Geometry check sheet. Reference: the model listing, model coordinates, mm. A direction names the side the tool comes from. Give positions to 0.01 mm unless a question says otherwise; leave off trailing zeros. Loops run counter-clockwise (first coordinate to the right, second up) from the corner with the lowest first, then second, coordinate; pieces in that order, holes last. Notation, with made-up numbers: (-8.5, 1.25) -> (4.5, 1.25) arc R20 ccw to (4.5, 31.25) -> close; hole circle Ø5 at (85.25, 18.25). An arc over 180 degrees is marked (long way). Answer as a JSON object with one key per item and string values.
Autodesk Inventor part; units mm, degrees
ref_plane "YZ Plane" through (0, 0, 0) normal (1, 0, 0) x (0, 1, 0)
ref_plane "XZ Plane" through (0, 0, 0) normal (0, 1, 0) x (-1, 0, 0)
ref_plane "XY Plane" through (0, 0, 0) normal (0, 0, 1) x (1, 0, 0)
sketch "Sketch2" plane through (0, 0, 0) normal (0, 0, 1) x (1, 0, 0)
  line L0 (-38.1, 105.1577) -> (50.8, 105.1577)
  line L1 (50.8, 105.1577) -> (50.8, 16.2577)
  line L2 (50.8, 16.2577) -> (-38.1, 16.2577)
  line L3 (-38.1, 16.2577) -> (-38.1, 105.1577)
  point P0 (0, 0)
  dimension "d45" = 88.9
  dimension "d46" = 88.9
extrude "Extrusion1" add sketch "Sketch2" along normal blind 2.54
sketch "Sketch3" plane through (0, 0, 0) normal (0, 0, -1) x (-1, 0, 0)
  circle A0 centre (-43.18, 97.5377) radius 4.0005
  line L0 (-50.8, 16.2577) -> (-50.8, 105.1577)
  line L1 (-50.8, 105.1577) -> (38.1, 105.1577)
  circle A1 centre (-43.18, 97.5377) radius 5.2705
  line L2 (38.1, 105.1577) -> (38.1, 16.2577)
  line L3 (38.1, 16.2577) -> (-50.8, 16.2577)
  circle A2 centre (-43.18, 84.8377) radius 5.2705
  circle A3 centre (-30.48, 97.5377) radius 5.2705
  circle A4 centre (-30.48, 84.8377) radius 5.2705
  circle A5 centre (-17.78, 97.5377) radius 5.2705
  circle A6 centre (-17.78, 84.8377) radius 5.2705
  line L4 (-45.1739, 77.2092) -> (-41.1861, 77.2092)
  line L5 (-41.1861, 77.2092) -> (-41.1861, 74.1358)
  line L6 (-41.1861, 74.1358) -> (-45.1739, 74.1358)
  line L7 (-45.1739, 74.1358) -> (-45.1739, 77.2092)
  line L8 (-45.1739, 77.2092) -> (-41.1861, 74.1358) construction
  line L9 (-41.1861, 77.2092) -> (-45.1739, 74.1358) construction
  line L10 (-45.9813, 73.5135) -> (-40.3787, 73.5135)
  line L11 (-40.3787, 73.5135) -> (-40.3787, 77.8315)
  line L12 (-40.3787, 77.8315) -> (-45.9813, 77.8315)
  line L13 (-45.9813, 77.8315) -> (-45.9813, 73.5135)
  line L14 (-45.9813, 73.5135) -> (-40.3787, 77.8315) construction
  line L15 (-40.3787, 73.5135) -> (-45.9813, 77.8315) construction
  circle A7 centre (-30.48, 97.5377) radius 4.1255
  circle A8 centre (-17.78, 97.5377) radius 4.2505
  circle A9 centre (-43.18, 84.8377) radius 4.3755
  circle A10 centre (-30.48, 84.8377) radius 4.5005
  circle A11 centre (-17.78, 84.8377) radius 4.6255
  line L16 (-32.7587, 77.8315) -> (-38.3613, 77.8315)
  line L17 (-38.3613, 77.8315) -> (-38.3613, 73.5135)
  line L18 (-38.3613, 73.5135) -> (-32.7587, 73.5135)
  line L19 (-32.7587, 73.5135) -> (-32.7587, 77.8315)
  line L20 (-25.1387, 77.8315) -> (-30.7413, 77.8315)
  line L21 (-30.7413, 77.8315) -> (-30.7413, 73.5135)
  line L22 (-30.7413, 73.5135) -> (-25.1387, 73.5135)
  line L23 (-25.1387, 73.5135) -> (-25.1387, 77.8315)
  line L24 (-17.5187, 77.8315) -> (-23.1213, 77.8315)
  line L25 (-23.1213, 77.8315) -> (-23.1213, 73.5135)
  line L26 (-23.1213, 73.5135) -> (-17.5187, 73.5135)
  line L27 (-17.5187, 73.5135) -> (-17.5187, 77.8315)
  line L28 (-9.8987, 77.8315) -> (-15.5013, 77.8315)
  line L29 (-15.5013, 77.8315) -> (-15.5013, 73.5135)
  line L30 (-15.5013, 73.5135) -> (-9.8987, 73.5135)
  line L31 (-9.8987, 73.5135) -> (-9.8987, 77.8315)
  line L32 (-37.6789, 74.0108) -> (-33.4411, 74.0108)
  line L33 (-33.4411, 74.0108) -> (-33.4411, 77.3342)
  line L34 (-33.4411, 77.3342) -> (-37.6789, 77.3342)
  line L35 (-37.6789, 77.3342) -> (-37.6789, 74.0108)
  line L36 (-37.6789, 74.0108) -> (-33.4411, 77.3342) construction
  line L37 (-33.4411, 74.0108) -> (-37.6789, 77.3342) construction
  line L38 (-30.1839, 73.8858) -> (-25.6961, 73.8858)
  line L39 (-25.6961, 73.8858) -> (-25.6961, 77.4592)
  line L40 (-25.6961, 77.4592) -> (-30.1839, 77.4592)
  line L41 (-30.1839, 77.4592) -> (-30.1839, 73.8858)
  line L42 (-30.1839, 73.8858) -> (-25.6961, 77.4592) construction
  line L43 (-25.6961, 73.8858) -> (-30.1839, 77.4592) construction
  line L44 (-22.6889, 73.7608) -> (-17.9511, 73.7608)
  line L45 (-17.9511, 73.7608) -> (-17.9511, 77.5842)
  line L46 (-17.9511, 77.5842) -> (-22.6889, 77.5842)
  line L47 (-22.6889, 77.5842) -> (-22.6889, 73.7608)
  line L48 (-22.6889, 73.7608) -> (-17.9511, 77.5842) construction
  line L49 (-17.9511, 73.7608) -> (-22.6889, 77.5842) construction
  line L50 (-45.1739, 73.4552) -> (-41.1861, 73.4552)
  line L51 (-41.1861, 73.4552) -> (-41.1861, 74.8164)
  line L52 (-41.1861, 74.8164) -> (-45.1739, 74.8164)
  line L53 (-45.1739, 74.8164) -> (-45.1739, 73.4552)
  line L54 (-45.1739, 73.4552) -> (-41.1861, 74.8164) construction
  line L55 (-41.1861, 73.4552) -> (-45.1739, 74.8164) construction
  point P0 (0, 0)
  point P1 (-43.18, 75.6725)
  point P2 (-43.18, 75.6725)
  point P3 (-35.56, 75.6725)
  point P4 (-27.94, 75.6725)
  point P5 (-20.32, 75.6725)
  point P6 (-12.7, 75.6725)
  point P7 (-43.18, 74.1358)
  dimension "d49" = 7.62
  dimension "d50" = 7.62
  dimension "d51" = 1.27
  dimension "d56" = 12.7
  dimension "d59" = 12.7
  dimension "d64" = 3.9878
  dimension "d65" = 3.0734
  dimension "d66" = 9.1652
  dimension "d67" = 2.159
  dimension "d77" = 8.001
  dimension "d78" = 8.251
  dimension "d80" = 8.501
  dimension "d81" = 8.751
  dimension "d82" = 9.001
  dimension "d83" = 9.251
  dimension "d90" = 7.62
  dimension "d95" = 4.2378
  dimension "d96" = 4.4878
  dimension "d97" = 4.7378
  dimension "d98" = 3.3234
  dimension "d99" = 3.5734
sketch "Sketch4" plane through (0, 0, 0) normal (0, 0, -1) x (-1, 0, 0)
  line L0 (-50.8, 105.1577) -> (38.1, 105.1577)
  line L1 (-50.8, 16.2577) -> (-50.8, 105.1577)
  line L2 (-50.8, 105.1577) -> (-48.5295, 105.1577)
  line L3 (-48.5295, 105.1577) -> (-48.5295, 103.1024)
  line L4 (-48.5295, 103.1024) -> (-50.8, 103.1024)
  line L5 (-50.8, 103.1024) -> (-50.8, 105.1577)
  point P0 (0, 0)
extrude "Extrusion4" cut sketch "Sketch3" against normal blind 9.001 contours A0 | A7 | A8 | A9 | A10 | A11
sketch "Sketch5" plane through (0, 0, 0) normal (0, 0, -1) x (-1, 0, 0)
  line L0 (-45.1739, 39.1092) -> (-41.1861, 39.1092)
  line L1 (-41.1861, 39.1092) -> (-41.1861, 36.0358)
  line L2 (-41.1861, 36.0358) -> (-45.1739, 36.0358)
  line L3 (-45.1739, 36.0358) -> (-45.1739, 39.1092)
  line L4 (-45.1739, 39.1092) -> (-41.1861, 36.0358) construction
  line L5 (-41.1861, 39.1092) -> (-45.1739, 36.0358) construction
  line L6 (-45.9813, 35.4135) -> (-40.3787, 35.4135)
  line L7 (-40.3787, 35.4135) -> (-40.3787, 39.7315)
  line L8 (-40.3787, 39.7315) -> (-45.9813, 39.7315)
  line L9 (-45.9813, 39.7315) -> (-45.9813, 35.4135)
  line L10 (-45.9813, 35.4135) -> (-40.3787, 39.7315) construction
  line L11 (-40.3787, 35.4135) -> (-45.9813, 39.7315) construction
  line L12 (-32.7587, 39.7315) -> (-38.3613, 39.7315)
  line L13 (-38.3613, 39.7315) -> (-38.3613, 35.4135)
  line L14 (-38.3613, 35.4135) -> (-32.7587, 35.4135)
  line L15 (-32.7587, 35.4135) -> (-32.7587, 39.7315)
  line L16 (-25.1387, 39.7315) -> (-30.7413, 39.7315)
  line L17 (-30.7413, 39.7315) -> (-30.7413, 35.4135)
  line L18 (-30.7413, 35.4135) -> (-25.1387, 35.4135)
  line L19 (-25.1387, 35.4135) -> (-25.1387, 39.7315)
  line L20 (-17.5187, 39.7315) -> (-23.1213, 39.7315)
  line L21 (-23.1213, 39.7315) -> (-23.1213, 35.4135)
  line L22 (-23.1213, 35.4135) -> (-17.5187, 35.4135)
  line L23 (-17.5187, 35.4135) -> (-17.5187, 39.7315)
  line L24 (-9.8987, 39.7315) -> (-15.5013, 39.7315)
  line L25 (-15.5013, 39.7315) -> (-15.5013, 35.4135)
  line L26 (-15.5013, 35.4135) -> (-9.8987, 35.4135)
  line L27 (-37.6789, 35.9108) -> (-33.4411, 35.9108)
  line L28 (-33.4411, 35.9108) -> (-33.4411, 39.2342)
  line L29 (-33.4411, 39.2342) -> (-37.6789, 39.2342)
  line L30 (-37.6789, 39.2342) -> (-37.6789, 35.9108)
  line L31 (-37.6789, 35.9108) -> (-33.4411, 39.2342) construction
  line L32 (-33.4411, 35.9108) -> (-37.6789, 39.2342) construction
  line L33 (-30.1839, 35.7858) -> (-25.6961, 35.7858)
  line L34 (-25.6961, 35.7858) -> (-25.6961, 39.3592)
  line L35 (-25.6961, 39.3592) -> (-30.1839, 39.3592)
  line L36 (-30.1839, 39.3592) -> (-30.1839, 35.7858)
  line L37 (-30.1839, 35.7858) -> (-25.6961, 39.3592) construction
  line L38 (-25.6961, 35.7858) -> (-30.1839, 39.3592) construction
  line L39 (-22.6889, 35.6608) -> (-17.9511, 35.6608)
  line L40 (-17.9511, 35.6608) -> (-17.9511, 39.4842)
  line L41 (-17.9511, 39.4842) -> (-22.6889, 39.4842)
  line L42 (-22.6889, 39.4842) -> (-22.6889, 35.6608)
  line L43 (-22.6889, 35.6608) -> (-17.9511, 39.4842) construction
  line L44 (-17.9511, 35.6608) -> (-22.6889, 39.4842) construction
  line L45 (-45.1516, 35.2931) -> (-41.1861, 36.7869) construction
  line L46 (-41.1861, 35.3552) -> (-45.1739, 36.7164) construction
  line L47 (-44.9867, 35.3552) -> (-41.3733, 35.3552)
  line L48 (-41.3733, 35.3552) -> (-41.3733, 36.7164)
  line L49 (-41.3733, 36.7164) -> (-44.9867, 36.7164)
  line L50 (-44.9867, 36.7164) -> (-44.9867, 35.3552)
  line L51 (-44.9867, 35.3552) -> (-41.3733, 36.7164) construction
  line L52 (-41.3733, 35.3552) -> (-44.9867, 36.7164) construction
  line L53 (-37.5427, 35.3747) -> (-33.5773, 35.3747)
  line L54 (-33.5773, 35.3747) -> (-33.5773, 36.447)
  line L55 (-33.5773, 36.447) -> (-37.5427, 36.447)
  line L56 (-37.5427, 36.447) -> (-37.5427, 35.3747)
  line L57 (-37.5427, 35.3747) -> (-33.5773, 36.447) construction
  line L58 (-33.5773, 35.3747) -> (-37.5427, 36.447) construction
  line L59 (-30.0124, 35.3468) -> (-25.8676, 35.3468)
  line L60 (-25.8676, 35.3468) -> (-25.8676, 36.2248)
  line L61 (-25.8676, 36.2248) -> (-30.0124, 36.2248)
  line L62 (-30.0124, 36.2248) -> (-30.0124, 35.3468)
  line L63 (-30.0124, 35.3468) -> (-25.8676, 36.2248) construction
  line L64 (-25.8676, 35.3468) -> (-30.0124, 36.2248) construction
  line L65 (-22.4558, 35.2013) -> (-18.1842, 35.2013)
  line L66 (-18.1842, 35.2013) -> (-18.1842, 36.1203)
  line L67 (-18.1842, 36.1203) -> (-22.4558, 36.1203)
  line L68 (-22.4558, 36.1203) -> (-22.4558, 35.2013)
  line L69 (-22.4558, 35.2013) -> (-18.1842, 36.1203) construction
  line L70 (-18.1842, 35.2013) -> (-22.4558, 36.1203) construction
  point P0 (0, 0)
  point P1 (-43.18, 37.5725)
  point P2 (-43.18, 37.5725)
  point P3 (-35.56, 37.5725)
  point P4 (-27.94, 37.5725)
  point P5 (-20.32, 37.5725)
  point P6 (-12.7, 37.5725)
  point P7 (-43.18, 36.0358)
  point P8 (-35.56, 35.9108)
  point P9 (-27.94, 35.7858)
  point P10 (-20.32, 35.6608)
  point P11 (-22.4558, 35.4135)
  point P12 (-22.4558, 35.6608)
  point P13 (-18.1842, 35.6608)
  point P14 (-18.1842, 35.4135)
  point P15 (-30.0124, 35.4135)
  point P16 (-30.0124, 35.7858)
  point P17 (-25.8676, 35.7858)
  point P18 (-25.8676, 35.4135)
  point P19 (-37.5427, 35.4135)
  point P20 (-37.5427, 35.9108)
  point P21 (-33.5773, 35.9108)
  point P22 (-33.5773, 35.4135)
  point P23 (-44.9867, 35.4135)
  point P24 (-44.9867, 36.0358)
  point P25 (-41.3733, 36.0358)
  point P26 (-41.3733, 35.4135)
  dimension "d102" = 3.0734
  dimension "d103" = 2.159
  dimension "d104" = 7.62
  dimension "d105" = 4.2378
  dimension "d106" = 4.4878
  dimension "d107" = 4.7378
  dimension "d108" = 3.3234
  dimension "d109" = 3.5734
extrude "Extrusion5" add sketch "Sketch5" along normal blind 2.54 contours L3 L2 L50 L6 L9 L8 L7 L48 L1 L0 | L15 L14 L54 L27 L28 L29 L30 L56 L13 L12 | L19 L18 L60 L33 L34 L35 L36 L62 L17 L16 | L23 L22 L66 L39 L40 L41 L42 L68 L21 L20
sketch "Sketch6" plane through (0, 0, 0) normal (0, 0, -1) x (-1, 0, 0)
  line L0 (-52.3953, 34.0161) -> (-4.7261, 34.0161)
  line L1 (-4.7261, 34.0161) -> (-4.7261, 12.2528)
  line L2 (-4.7261, 12.2528) -> (-52.3953, 12.2528)
  line L3 (-52.3953, 12.2528) -> (-52.3953, 34.0161)
  point P0 (0, 0)
extrude "Extrusion6" cut sketch "Sketch6" against normal blind 2.54
sketch "Sketch7" plane through (0, 0, 0) normal (0, 0, -1) x (-1, 0, 0)
  point P0 (0, 0)
equation "\"d86\" = d82"
properties part number "magnet_hall_testing_w_trucks"
1) Tool access check on faces 3 (the face through (17.519, 38, -1)), 4 (the face through (30.184, 38, -1)), 5 (the face through (25.139, 38, -1)), 6 (the face through (43.6, 39.3, -2.54)), 7 (the face through (43.701, 101.504, 1.252)). Record the directions out of +Z, -Z, +X, -X, +Y, -Y that give a thin tool (end or side, any length) a straight path to the whole face; none if there is none.
Geometry check:
{"face 3": "-Z, -X, +Y, -Y", "face 4": "-Z", "face 5": "-Z, +Y, -Y", "face 6": "-Z, +X, -X, +Y, -Y", "face 7": "+Z, -Z"}
2) Section check D-D on y = 77.5. Record the cut outline in (x, z), plus the area to 3 significant figures.
Geometry check:
{"outline": "(-38.1, 0) -> (50.8, 0) -> (50.8, 2.54) -> (-38.1, 2.54) -> close", "area": "226 mm2"}
3) Draft check along Y on faces 1 (the face through (33.441, 38, -1)), 2 (the face through (45.981, 38, -1)). Enter one of: pulls with the +Y half, pulls with the -Y half, needs draft (parallel to the pull), parting line crosses it, or undercut.
Geometry check:
{"face 1": "undercut", "face 2": "needs draft"}
4) Depth check by flat-ended pin: P1, Ø1.3, axis at y = 38, z = -1, coming from the +X side; P2, Ø2, axis at y = 62.5, z = -1.5, coming from the +X side; P3, Ø8, axis at x = -11.5, y = 78.5, coming from the -Z side; P4, Ø1.3, axis at y = 38, z = -1, coming from the -X side. Enter the tip coordinate at first touch or a pass-through.
Geometry check:
{"P1": "stops at x = 45.98", "P2": "passes through", "P3": "stops at z = 0", "P4": "stops at x = 17.52"}
5) Material ranges on line 1 along Y through (x, z) = (43.18, 0.85); line 2 along Y through (x, z) = (30.48, 2); line 3 along X through (y, z) = (96, 1.3), recorded low to high. Write a range as from..to.
Geometry check:
{"line 1": "y = 34.02..80.46, 89.21..93.54, 101.54..105.16", "line 2": "y = 34.02..80.34, 89.34..93.41, 101.66..105.16", "line 3": "x = -38.1..13.82, 21.74..26.65, 34.31..39.49, 46.87..50.8"}
6) Section check A-A on x = 43.18. Record the cut outline in (y, z), plus the area to 3 significant figures.
Geometry check:
{"outline": "(34.02, 0) -> (39.11, 0) -> (39.11, -2.54) -> (39.73, -2.54) -> (39.73, 0) -> (80.46, 0) -> (80.46, 2.54) -> (34.02, 2.54) -> close; (89.21, 0) -> (93.54, 0) -> (93.54, 2.54) -> (89.21, 2.54) -> close; (101.54, 0) -> (105.16, 0) -> (105.16, 2.54) -> (101.54, 2.54) -> close", "area": "140 mm2"}
7) Section check B-B on z = -0.9. Count the separate pieces of the cut face and the enclosed holes in it, plus the area to 3 significant figures.
Geometry check:
{"separate pieces": "4", "enclosed holes": "0", "area": "29.5 mm2"}
8) Section check C-C on x = 21. Record the cut outline in (y, z), plus the area to 3 significant figures.
Geometry check:
{"outline": "(34.02, 0) -> (39.48, 0) -> (39.48, -2.54) -> (39.73, -2.54) -> (39.73, 0) -> (81.52, 0) -> (81.52, 2.54) -> (34.02, 2.54) -> close; (88.16, 0) -> (94.76, 0) -> (94.76, 2.54) -> (88.16, 2.54) -> close; (100.31, 0) -> (105.16, 0) -> (105.16, 2.54) -> (100.31, 2.54) -> close", "area": "150 mm2"}
